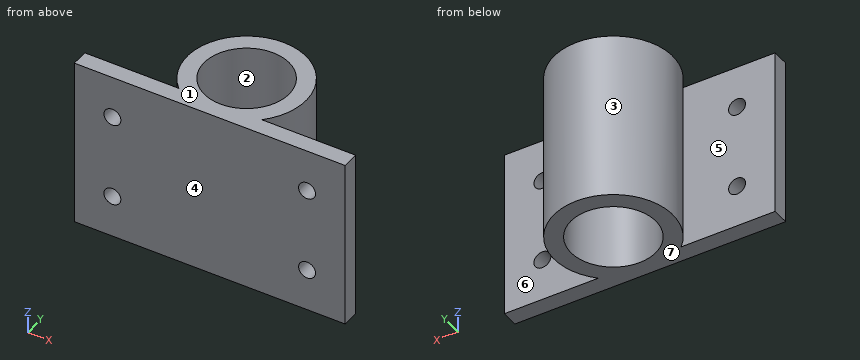
from build123d import *

# Parameters (mm, degrees)
SKETCH2_R           = 25
BOSS_EXTRUDE1_DEPTH = 100
SKETCH3_R           = 5
CUT_EXTRUDE1_DEPTH  = 10


with BuildPart() as part:
    # Sketch2 → Boss-Extrude1 (new body)
    with BuildSketch(Plane.XY):
        with BuildLine():
            Line((-80, -35), (80, -35))
            Line((80, -35), (80, -25))
            Line((80, -25), (24.494897428, -25))
            ThreePointArc((24.494897428, -25), (0, 35), (-24.494897428, -25))
            Line((-24.494897428, -25), (-80, -25))
            Line((-80, -25), (-80, -35))
        make_face()
        Circle(SKETCH2_R, mode=Mode.SUBTRACT)
    extrude(amount=BOSS_EXTRUDE1_DEPTH)

    # Sketch3 → Cut-Extrude1 (cut)
    with BuildSketch(Plane(origin=(0, -25, 0), x_dir=(1, 0, 0), z_dir=(0, 1, 0))):
        with Locations(Location((57.5, -25, 0), (0, 0, 180))):
            Circle(SKETCH3_R)
        with Locations(Location((57.5, -75, 0), (0, 0, 180))):
            Circle(SKETCH3_R)
        with Locations(Location((-57.5, -25, 0), (0, 0, 180))):
            Circle(SKETCH3_R)
        with Locations(Location((-57.5, -75, 0), (0, 0, 180))):
            Circle(SKETCH3_R)
    extrude(amount=-CUT_EXTRUDE1_DEPTH, mode=Mode.SUBTRACT)


solid = part.part
CAD build for the part. Positions are in the model's coordinates, mm. Face numbers are marked on the shaded views. A direction names the side the tool comes from. Round coordinates to 2 decimals unless told otherwise and drop trailing zeros. Loops run counter-clockwise (first coordinate to the right, second up) from the corner with the lowest first, then second, coordinate; pieces in that order, holes last.
(1) Cut at B-B (x = 57.5). Give the cut face in (y, z).
(2) Cut at C-C (y = 0). Give the cut face in (x, z), plus the area to 3 significant figures.
(3) Drop flat-ended pins along their axis: pin 1 (4 mm diameter, centred on y = 10, z = 60, fed in from +X); pin 2 (12 mm diameter, centred on y = 10, z = 85.5, fed in from +X); pin 3 (16 mm diameter, centred on x = -57.5, z = 75, fed in from +Y). Give the stop position or say it passes through.
(4) Two-plate mould, pull along Y, no slides. Class the marked faces 1, 2, 3 and 4: +Y half, -Y half, draft (parallel to the pull), parting line (faces both ways), or undercut.
(5) Which spindle directions (+Z, -Z, +X, -X, +Y, -Y) get a long thin tool onto all of the face, cutting with end or side? Do the marked faces 5, 6 and 7. Say none if no direction does.
(6) Cut at A-A (z = 75). Give the cut face in (x, y), plus the area to 3 significant figures.
(7) Wall check: line 1 along Z through (x, y) = (-57.5, -31); line 2 along X through (y, z) = (1, 95); line 3 along Y through (x, z) = (54, 40). Give the ranges that are in metal, low to high.
Findings below:
1. outline: (-35, 0) - (-25, 0) - (-25, 20) - (-35, 20) - close; (-35, 30) - (-25, 30) - (-25, 70) - (-35, 70) - close; (-35, 80) - (-25, 80) - (-25, 100) - (-35, 100) - close
2. outline: (-35, 0) - (-25, 0) - (-25, 100) - (-35, 100) - close; (25, 0) - (35, 0) - (35, 100) - (25, 100) - close
2. area: 2,000 mm2
3. pin 1: stops at x = 34.07
3. pin 2: stops at x = 34.77
3. pin 3: stops at y = -25
4. face 1: draft
4. face 2: undercut
4. face 3: undercut
4. face 4: -Y half
5. face 5: +Z, -Z, -X
5. face 6: +Z, -Z, +X
5. face 7: -Z, +X, -X, +Y, -Y
6. outline: (-80, -35) - (-62.5, -35) - (-62.5, -25) - (-80, -25) - close; (-52.5, -35) - (52.5, -35) - (52.5, -25) - (24.49, -25) arc R35 ccw (long way) to (-24.49, -25) - (-52.5, -25) - close; (62.5, -35) - (80, -35) - (80, -25) - (62.5, -25) - close; hole circle Ø50 at (0, 0)
6. area: 2,950 mm2
7. line 1: z = 0 to 20, 30 to 70, 80 to 100
7. line 2: x = -34.99 to -24.98, 24.98 to 34.99
7. line 3: y = -35 to -25
